Check sheet for the modelled part. Datum: model origin and axes. Units: mm. Face numbers are marked on the shaded views. A direction names the side the tool comes from. Round coordinates to 2 decimals unless told otherwise and drop trailing zeros. Loops run counter-clockwise (first coordinate to the right, second up) from the corner with the lowest first, then second, coordinate; pieces in that order, holes last. Notation, with made-up numbers: (17.5, 2.5) -> (68.5, 2.5) arc R31 ccw to (68.5, 32.5) -> close; hole circle Ø1 at (-7.5, -17.75). An arc over 180 degrees is marked (long way). Return JSON: item names as keys, results as strings.
Autodesk Inventor part; units mm, degrees
ref_plane "YZ Plane" through (0, 0, 0) normal (1, 0, 0) x (0, 1, 0)
ref_plane "XZ Plane" through (0, 0, 0) normal (0, 1, 0) x (-1, 0, 0)
ref_plane "XY Plane" through (0, 0, 0) normal (0, 0, 1) x (1, 0, 0)
sketch "Sketch1" plane through (0, 0, 0) normal (0, 1, 0) x (-1, 0, 0)
  line L0 (-2.85, 1.9) -> (2.85, 1.9)
  line L1 (2.85, 1.9) -> (2.85, -1.9)
  line L2 (2.85, -1.9) -> (-2.85, -1.9)
  line L3 (-2.85, -1.9) -> (-2.85, 1.9)
  line L4 (-2.85, 1.9) -> (2.85, -1.9) construction
  line L5 (2.85, 1.9) -> (-2.85, -1.9) construction
  line L6 (3.45, -2.5) -> (3.45, 2.5)
  line L7 (3.45, 2.5) -> (-3.45, 2.5)
  line L8 (-3.45, 2.5) -> (-3.45, -2.5)
  line L9 (-3.45, -2.5) -> (3.45, -2.5)
  circle A0 centre (0, 0) radius 2.85
  circle A1 centre (0, 0) radius 3.45
  point P0 (-2.1243, 1.9)
  point P1 (2.1243, 1.9)
  point P2 (2.1243, -1.9)
  point P3 (-2.1243, -1.9)
  point P4 (-2.3775, 2.5)
  point P5 (-2.3775, -2.5)
  point P6 (2.3775, -2.5)
  point P7 (2.3775, 2.5)
  dimension "d0" = 3.8
  dimension "d1" = 0.6
  dimension "d2" = 5.7
extrude "Extrusion1" add sketch "Sketch1" along normal blind 7.5 contours L3 L2 A0 L9 A1 L7 L0 | L0 A0 L3 | A0 L7 L0 | A0 L2 L3 | A0 L7 A1 L9 L2 L1 L0 | L0 L1 A0 | L2 A0 L9 | L1 L2 A0
sketch "Sketch2" plane through (0, 7.5, 0) normal (0, 1, 0) x (1, 0, 0)
  arc A0 (2.3775, -2.5) -> (2.3775, 2.5) centre (0, 0) ccw
  line L0 (2.3775, 2.5) -> (-2.3775, 2.5)
  arc A1 (-2.3775, 2.5) -> (-2.3775, -2.5) centre (0, 0) ccw
  line L1 (-2.3775, -2.5) -> (2.3775, -2.5)
  arc A2 (2.1243, -1.9) -> (2.1243, 1.9) centre (0, 0) ccw
  line L2 (2.1243, -1.9) -> (-2.1243, -1.9)
  arc A3 (-2.1243, 1.9) -> (-2.1243, -1.9) centre (0, 0) ccw
  line L3 (-2.1243, 1.9) -> (2.1243, 1.9)
extrude "Extrusion2" add sketch "Sketch2" along normal blind 0.5 contours L1 A1 L0 A0 | L2 A3 L3 A2
sketch "Sketch3" plane through (0, 8, 0) normal (0, 1, 0) x (1, 0, 0)
  line L0 (-0.925, -2.625) -> (-0.925, 2.625)
  line L1 (-0.925, 2.625) -> (0.925, 2.625)
  line L2 (0.925, 2.625) -> (0.925, -2.625)
  line L3 (0.925, -2.625) -> (-0.925, -2.625)
  line L4 (-0.925, -2.625) -> (0.925, 2.625) construction
  line L5 (-0.925, 2.625) -> (0.925, -2.625) construction
  line L6 (-2.625, -0.925) -> (2.625, -0.925)
  line L7 (2.625, -0.925) -> (2.625, 0.925)
  line L8 (2.625, 0.925) -> (-2.625, 0.925)
  line L9 (-2.625, 0.925) -> (-2.625, -0.925)
  line L10 (-2.625, -0.925) -> (2.625, 0.925) construction
  line L11 (2.625, -0.925) -> (-2.625, 0.925) construction
  line L12 (-3.125, 1.425) -> (3.125, 1.425)
  line L13 (3.125, 1.425) -> (3.125, -1.425)
  line L14 (3.125, -1.425) -> (-3.125, -1.425)
  line L15 (-3.125, -1.425) -> (-3.125, 1.425)
  line L16 (1.425, -3.125) -> (1.425, 3.125)
  line L17 (1.425, 3.125) -> (-1.425, 3.125)
  line L18 (-1.425, 3.125) -> (-1.425, -3.125)
  line L19 (-1.425, -3.125) -> (1.425, -3.125)
  point P0 (0, 0)
  point P1 (-1.425, -1.425)
  point P2 (1.425, -1.425)
  point P3 (1.425, 1.425)
  point P4 (-1.425, 1.425)
  dimension "d7" = 5.25
  dimension "d8" = 5.25
  dimension "d9" = 1.85
  dimension "d10" = 1.85
  dimension "d11" = 0.5
  dimension "d12" = 0.5
extrude "Extrusion3" add sketch "Sketch3" along normal blind 0.5
sketch "Sketch4" plane through (0, 8.5, 0) normal (0, 1, 0) x (1, 0, 0)
  line L0 (-3.125, 1.425) -> (-3.125, -1.425)
  line L1 (-3.125, -1.425) -> (-1.425, -1.425)
  line L2 (-1.425, -1.425) -> (-1.425, -3.125)
  line L3 (-1.425, -3.125) -> (1.425, -3.125)
  line L4 (1.425, -3.125) -> (1.425, -1.425)
  line L5 (1.425, -1.425) -> (3.125, -1.425)
  line L6 (3.125, -1.425) -> (3.125, 1.425)
  line L7 (3.125, 1.425) -> (1.425, 1.425)
  line L8 (1.425, 1.425) -> (1.425, 3.125)
  line L9 (1.425, 3.125) -> (-1.425, 3.125)
  line L10 (-1.425, 3.125) -> (-1.425, 1.425)
  line L11 (-1.425, 1.425) -> (-3.125, 1.425)
  line L12 (-2.625, -0.925) -> (-2.625, 0.925)
  line L13 (-2.625, 0.925) -> (-0.925, 0.925)
  line L14 (-0.925, 0.925) -> (-0.925, 2.625)
  line L15 (-0.925, 2.625) -> (0.925, 2.625)
  line L16 (0.925, 2.625) -> (0.925, 0.925)
  line L17 (0.925, 0.925) -> (2.625, 0.925)
  line L18 (2.625, 0.925) -> (2.625, -0.925)
  line L19 (2.625, -0.925) -> (0.925, -0.925)
  line L20 (0.925, -0.925) -> (0.925, -2.625)
  line L21 (0.925, -2.625) -> (-0.925, -2.625)
  line L22 (-0.925, -2.625) -> (-0.925, -0.925)
  line L23 (-0.925, -0.925) -> (-2.625, -0.925)
  point P0 (0, 0)
  dimension "d15" = 0.5
extrude "Extrusion4" add sketch "Sketch4" along normal blind 6
fillet "Fillet1" radius 0.3 8 edges at (1.425, 11.25, 3.125) (3.125, 11.25, 1.425) (3.125, 11.25, -1.425) (1.425, 11.25, -3.125) (-1.425, 11.25, -3.125) (-3.125, 11.25, -1.425) (-1.425, 11.25, 3.125) (-3.125, 11.25, 1.425)
fillet "Fillet2" radius 0.3 4 edges at (-0.925, 11.5, 0.925) (0.925, 11.5, 0.925) (0.925, 11.5, -0.925) (-0.925, 11.5, -0.925)
fillet "Fillet3" radius 0.5 4 edges at (2.3775, 4, -2.5) (-2.3775, 4, -2.5) (-2.3775, 4, 2.5) (2.3775, 4, 2.5)
sketch "Sketch5" plane through (0, 8.5, 0) normal (0, 1, 0) x (1, 0, 0)
  line L0 (2.625, 0.925) -> (1.225, 0.925)
  arc A0 (0.925, 1.225) -> (1.225, 0.925) centre (1.225, 1.225) ccw
  line L1 (0.925, 1.225) -> (0.925, 2.625)
  line L2 (0.925, 2.625) -> (-0.925, 2.625)
  line L3 (-0.925, 2.625) -> (-0.925, 1.225)
  arc A1 (-1.225, 0.925) -> (-0.925, 1.225) centre (-1.225, 1.225) ccw
  line L4 (-1.225, 0.925) -> (-2.625, 0.925)
  line L5 (-2.625, 0.925) -> (-2.625, -0.925)
  line L6 (-2.625, -0.925) -> (-1.225, -0.925)
  arc A2 (-0.925, -1.225) -> (-1.225, -0.925) centre (-1.225, -1.225) ccw
  line L7 (-0.925, -1.225) -> (-0.925, -2.625)
  line L8 (-0.925, -2.625) -> (0.925, -2.625)
  line L9 (0.925, -2.625) -> (0.925, -1.225)
  arc A3 (1.225, -0.925) -> (0.925, -1.225) centre (1.225, -1.225) ccw
  line L10 (1.225, -0.925) -> (2.625, -0.925)
  line L11 (2.625, -0.925) -> (2.625, 0.925)
  line L12 (-2.1243, 1.9) -> (2.1243, 1.9)
  arc A4 (2.1243, -1.9) -> (2.1243, 1.9) centre (0, 0) ccw
  line L13 (2.1243, -1.9) -> (-2.1243, -1.9)
  arc A5 (-2.1243, 1.9) -> (-2.1243, -1.9) centre (0, 0) ccw
  point P0 (2.5898, -0.925)
  point P1 (2.625, -0.8197)
  point P2 (2.625, 0.8197)
  point P3 (2.5898, 0.925)
  point P4 (0.925, 1.9)
  point P5 (-0.925, 1.9)
  point P6 (-2.5898, 0.925)
  point P7 (-2.625, 0.8197)
  point P8 (-2.625, -0.8197)
  point P9 (-2.5898, -0.925)
  point P10 (-0.925, -1.9)
  point P11 (0.925, -1.9)
extrude "Extrusion5" cut sketch "Sketch5" against normal up to surface (1 mm away) contours L11 L10 A3 L9 L13 L7 A2 L6 L5 L4 A1 L3 L12 L1 A0 L0
fillet "Fillet4" radius 0.2 4 edges at (-1.425, 11.25, 1.425) (1.425, 11.25, 1.425) (1.425, 11.25, -1.425) (-1.425, 11.25, -1.425)
equation "\"d8\" = d7"
equation "\"d10\" = d9"
equation "\"d12\" = d11"
equation "\"d15\" = d11"
properties part number "motor-lego-adapter-3-4"
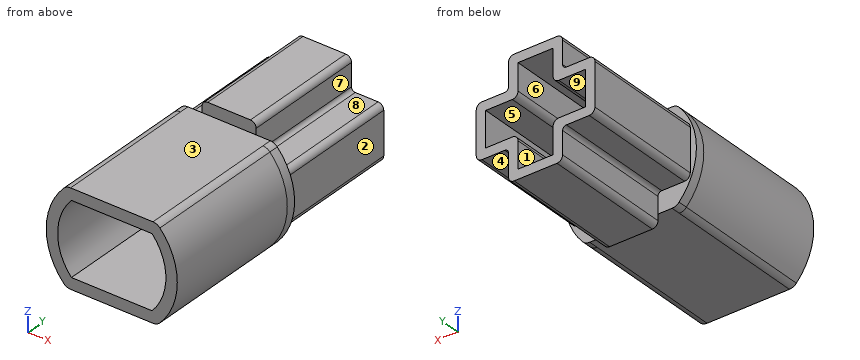
Q1. Section check B-B (y = 2). Record the boundary of the cut face in (x, z).
Results list:
{"outline": "(-2.54, -2.34) arc R0.5 ccw to (-2.17, -2.5) -> (2.17, -2.5) arc R0.5 ccw to (2.54, -2.34) arc R3.45 ccw to (2.54, 2.34) arc R0.5 ccw to (2.17, 2.5) -> (-2.17, 2.5) arc R0.5 ccw to (-2.54, 2.34) arc R3.45 ccw to start; hole (-2.12, -1.9) -> (2.12, -1.9) arc R2.85 ccw to (2.12, 1.9) -> (-2.12, 1.9) arc R2.85 ccw to start"}
Q2. Go/stop test with flat-tipped pins: pin 1 (1.5 mm diameter, centred on y = 9.5, z = 1.5, fed in from +X) (3 decimals); pin 2 (1.5 mm diameter, centred on x = -1.5, y = 7, fed in from +Z); pin 3 (0.7 mm diameter, centred on y = 10.5, z = 0, fed in from -X) (3 decimals). Record where each tip stops, or that it passes through.
Results list:
{"pin 1": "x = 3.125", "pin 2": "z = 2.5", "pin 3": "x = -3.125"}
Q3. Material ranges on line 1 (Z direction, x = -0.5, y = 2.5); line 2 (X direction, y = 11, z = -1.75) (3 decimals), recorded low to high.
Results list:
{"line 1": "-2.5 to -1.9, 1.9 to 2.5", "line 2": "-1.425 to -0.925, 0.925 to 1.425"}
Q4. Section check A-A (x = 0). Record the boundary of the cut face in (y, z) (3 decimals), then the cut area to 3 significant figures.
Results list:
{"outline": "(0, -2.5) -> (8, -2.5) -> (8, -3.125) -> (14.5, -3.125) -> (14.5, -2.625) -> (8.5, -2.625) -> (8.5, -1.9) -> (0, -1.9) -> close; (0, 1.9) -> (8.5, 1.9) -> (8.5, 2.625) -> (14.5, 2.625) -> (14.5, 3.125) -> (8, 3.125) -> (8, 2.5) -> (0, 2.5) -> close", "area": "16.8 mm^2"}
Q5. Tool access check on the marked faces 1, 2, 3, 4 and 5. Record the directions out of +Z, -Z, +X, -X, +Y, -Y that give a thin tool (end or side, any length) a straight path to the whole face; none if there is none.
Results list:
{"face 1": "+Y", "face 2": "+Z, -Z, +X, +Y", "face 3": "+Z, +X, -X, -Y", "face 4": "-Z, +X, +Y", "face 5": "+Y, -Y"}
Q6. Section check C-C (z = -0.25). Record the boundary of the cut face in (x, y) (3 decimals), then the cut area to 3 significant figures.
Results list:
{"outline": "(-3.441, 0) -> (-2.839, 0) -> (-2.839, 7.5) -> (-2.625, 7.5) -> (-2.625, 14.5) -> (-3.125, 14.5) -> (-3.125, 8) -> (-3.441, 8) -> close; (2.625, 7.5) -> (2.839, 7.5) -> (2.839, 0) -> (3.441, 0) -> (3.441, 8) -> (3.125, 8) -> (3.125, 14.5) -> (2.625, 14.5) -> close", "area": "16.3 mm^2"}
Q7. Draft check along Z on the marked faces 6, 7, 8 and 9. Enter one of: released by +Z, released by -Z, zero draft, split by the parting line, or undercut.
Results list:
{"face 6": "undercut", "face 7": "zero draft", "face 8": "released by +Z", "face 9": "undercut"}
